Verification items for the finished model (mm, model axes). Coordinates: 2 decimals unless noted, no trailing zeros. Order: outer loops, then holes, each group sorted by start corner. A loop starts at its lowest first (then second) coordinate and runs counter-clockwise, first axis right, second up. Notation, with made-up numbers: (6, 53) - (64, 53) arc R22 ccw to (64, 63) - close; hole circle Ø8 at (2, 73.5). An arc over 180 degrees is marked (long way). Answer as CSV lines item,"result". Start each with the question number.
1. Section check C-C (y = -6). Record the cut outline in (x, z), and give its area (3 significant figures).
2. Section check A-A (z = 2.5). Record the cut outline in (x, y), and give its area (3 significant figures).
3. Section check B-B (x = 0.5). Record the cut outline in (y, z).
4. Material ranges on L1, parallel to Y at x = 1.75, z = 67; L2, parallel to X at y = -12.25, z = 66; L3, parallel to Z at x = -0.75, y = -9.5, recorded low to high. Write a range as [from, to].
5. Go/stop test with flat-tipped pins: pin 1 (6 mm diameter, centred on y = -12.5, z = -35, fed in from -X); pin 2 (4 mm diameter, centred on y = -13.5, z = -72.5, fed in from +X); pin 3 (1.5 mm diameter, centred on x = -0.5, z = 43.5, fed in from +Y). Record where each tip stops, or that it passes through.
6. Section check D-D (z = -70). Record the cut outline in (x, y), and give its area (3 significant figures).
7. Mould release check, pull along Y, two halves, no side actions. Record for faces 1 (the flat face through (0, -27, 4)), 2 (the cylindrical face through (0.06, -3.82, 13.59)), 3 (the flat face through (0, -11, -50)), 4 (the flat face through (4, -6, 7)): pulls with the +Y half, pulls with the -Y half, needs draft (parallel to the pull), parting line crosses it, or undercut.
from build123d import *

# Parameters (mm, degrees)
F1_DEPTH = 2.5
F2_DEPTH = 4


# Not quite as in the source:
# - a feature names something its author has since deleted; it is built from what else it names


with BuildPart() as f1:
    # F0 (on Right) → F1 (new body, symmetric)
    with BuildSketch(Plane.YZ):
        with BuildLine():
            Line((-11, 102.1741141677), (-27, 102.1741141677))
            Line((-27, 102.1741141677), (-27, -97.8258858323))
            Line((-27, -97.8258858323), (-11, -97.8258858323))
            Line((-11, -97.8258858323), (-11, 0))
            Line((-11, 0), (-12, 0))
            Line((-12, 0), (-12, 8))
            ThreePointArc((-12, 8), (-11.7445626465, 9.7320508076), (-11, 11.3166247904))
            Line((-11, 11.3166247904), (-11, 102.1741141677))
        make_face()
        with BuildLine():
            Line((-11, 0), (-11, 11.3166247904))
            ThreePointArc((-11, 11.3166247904), (-11.7445626465, 9.7320508076), (-12, 8))
            Line((-12, 8), (-12, 0))
            Line((-12, 0), (-11, 0))
        make_face()
    extrude(amount=F1_DEPTH, both=True)

    # F0 (on Right) → F2 (join, symmetric)
    with BuildSketch(Plane.YZ):
        with BuildLine():
            ThreePointArc((0, 8), (-4.2679491924, 13.7445626465), (-11, 11.3166247904))
            Line((-11, 11.3166247904), (-11, 0))
            Line((-11, 0), (0, 0))
            Line((0, 0), (0, 8))
        make_face()
        with BuildLine():
            Line((-11, 0), (-11, 11.3166247904))
            ThreePointArc((-11, 11.3166247904), (-11.7445626465, 9.7320508076), (-12, 8))
            Line((-12, 8), (-12, 0))
            Line((-12, 0), (-11, 0))
        make_face()
    extrude(amount=F2_DEPTH, both=True)


solid = f1.part
Evaluation:
1,outline,"(-4, 0) - (4, 0) - (4, 14) - (-4, 14) - close"
1,area,"112 mm²"
2,outline,"(-4, -12) - (-2.5, -12) - (-2.5, -27) - (2.5, -27) - (2.5, -12) - (4, -12) - (4, 0) - (-4, 0) - close"
2,area,"171 mm²"
3,outline,"(-27, -97.83) - (-11, -97.83) - (-11, 0) - (0, 0) - (0, 8) arc R6 ccw to (-11, 11.32) - (-11, 102.17) - (-27, 102.17) - close"
4,L1,"y = [-27, -11]"
4,L2,"x = [-2.5, 2.5]"
4,L3,"z = [0, 12.87]"
5,pin 1,"stops at x = -2.5"
5,pin 2,"stops at x = 2.5"
5,pin 3,"stops at y = -11"
6,outline,"(-2.5, -27) - (2.5, -27) - (2.5, -11) - (-2.5, -11) - close"
6,area,"80.0 mm²"
7,face 1,"pulls with the -Y half"
7,face 2,"undercut"
7,face 3,"pulls with the +Y half"
7,face 4,"needs draft"
